from build123d import *

# Parameters (mm, degrees)
ESQUISSE1_W             = 90
ESQUISSE1_H             = 65
ESQUISSE1_R             = 7
ESQUISSE1_R_2           = 13
BOSS_EXTRU_1_DEPTH      = 8
ESQUISSE2_R             = 13
BOSS_EXTRU_2_DEPTH      = 3
ESQUISSE3_R             = 7
ESQUISSE3_R_2           = 1.5
ENL_V_MAT_EXTRU_1_DEPTH = 112.130553854
ESQUISSE4_R             = 8
ENL_V_MAT_EXTRU_2_DEPTH = 5.5
ESQUISSE5_W             = 45
ESQUISSE5_H             = 25
ENL_V_MAT_EXTRU_3_DEPTH = 112.30588484


with BuildPart() as part:
    # Esquisse1 → Boss.-Extru.1 (new body)
    with BuildSketch(Plane.XY):
        with Locations((45, 32.5)):
            Rectangle(ESQUISSE1_W, ESQUISSE1_H)
        with Locations((70, 20)):
            Circle(ESQUISSE1_R, mode=Mode.SUBTRACT)
        with Locations((17, 20)):
            Circle(ESQUISSE1_R_2, mode=Mode.SUBTRACT)
        with Locations((25, 48)):
            Circle(ESQUISSE1_R_2, mode=Mode.SUBTRACT)
    extrude(amount=BOSS_EXTRU_1_DEPTH)

    # Esquisse2 → Boss.-Extru.2 (add)
    with BuildSketch(Plane(origin=(0, 0, 0), x_dir=(-1, 0, 0), z_dir=(0, 0, -1))):
        with Locations((-17, 20)):
            Circle(ESQUISSE2_R)
    extrude(amount=-BOSS_EXTRU_2_DEPTH)

    # Esquisse3 → Enlèv. mat.-Extru.1 (cut, through all)
    with BuildSketch(Plane.XY.offset(3)):
        with Locations((17, 20)):
            Circle(ESQUISSE3_R)
        with Locations((27, 20)):
            Circle(ESQUISSE3_R_2)
        with Locations((17, 10)):
            Circle(ESQUISSE3_R_2)
        with Locations((7, 20)):
            Circle(ESQUISSE3_R_2)
        with Locations((17, 30)):
            Circle(ESQUISSE3_R_2)
    extrude(amount=-ENL_V_MAT_EXTRU_1_DEPTH, mode=Mode.SUBTRACT)

    # Esquisse4 → Enlèv. mat.-Extru.2 (cut)
    with BuildSketch(Plane.XY.offset(8)):
        with Locations((70, 20)):
            Circle(ESQUISSE4_R)
    extrude(amount=-ENL_V_MAT_EXTRU_2_DEPTH, mode=Mode.SUBTRACT)

    # Esquisse5 → Enlèv. mat.-Extru.3 (cut, through all)
    with BuildSketch(Plane.XY.offset(8)):
        with Locations((67.5, 52.5)):
            Rectangle(ESQUISSE5_W, ESQUISSE5_H)
    extrude(amount=-ENL_V_MAT_EXTRU_3_DEPTH, mode=Mode.SUBTRACT)


solid = part.part
Input: part model. Units: mm. Frame: model coordinates. A direction names the side the tool comes from. Give positions to 0.01 mm unless a question says otherwise; leave off trailing zeros. Write each loop counter-clockwise with the first axis right and the second up, starting at its lowest first coordinate (ties: lowest second). Pieces come first, ordered by that corner, then holes. Notation, with made-up numbers: M -2,72.5 L 18,72.5 A31 ccw 18,104.5 Z; hole C -34,35 d5. An arc over 180 degrees is marked long. Use one line per item in the form item = value.
1. Cut plane D-D on x = 27. Return loops of the section in (y, z).
Outcome:
outline = M 0,0 L 18.5,0 L 18.5,3 L 11.69,3 L 11.69,8 L 0,8 Z; M 21.5,0 L 35.15,0 L 35.15,8 L 28.31,8 L 28.31,3 L 21.5,3 Z; M 60.85,0 L 65,0 L 65,8 L 60.85,8 Z
2. Mould query, pull axis X, two halves, no side actions, for faces 4 (the face through (74, 14, 2.5)), 5 (the face through (22, 65, 4)), 6 (the face through (45, 52, 4)). Classes: released by +X, released by -X, zero draft, split by the parting line, or undercut.
Outcome:
face_4 = undercut
face_5 = zero draft
face_6 = released by +X
3. Ray query, L1, parallel to Y at x = 25, z = 2.5; L2, parallel to X at y = 48.5, z = 7.75; L3, parallel to Y at x = 27, z = 0.7. Return the intervals inside material, ascending.
Outcome:
L1 = 0 to 35, 61 to 65
L2 = 0 to 12.01, 37.99 to 45
L3 = 0 to 18.5, 21.5 to 35.15, 60.85 to 65
4. Reachability of faces 1 (the face through (44, 26, 8)), 2 (the face through (62, 20, 5)), 3 (the face through (67, 40, 4)) from +Z, -Z, +X, -X, +Y, -Y: full face, straight path, thin tool, end or side. Return the list, or none.
Outcome:
face_1 = +Z, +X, -X, +Y, -Y
face_2 = +Z
face_3 = +Z, -Z, +X, +Y
5. Cut plane C-C on y = 48. Return loops of the section in (x, z), and give its area (3 significant figures).
Outcome:
outline = M 0,0 L 12,0 L 12,8 L 0,8 Z; M 38,0 L 45,0 L 45,8 L 38,8 Z
area = 152 mm²
6. Cut plane A-A on z = 1. Return loops of the section in (x, y), and give its area (3 significant figures).
Outcome:
outline = M 0,0 L 90,0 L 90,40 L 45,40 L 45,65 L 0,65 Z; hole C 7,20 d3; hole C 17,20 d14; hole C 25,48 d26; hole C 17,10 d3; hole C 17,30 d3; hole C 27,20 d3; hole C 70,20 d14
area = 3,860 mm²
7. Cut plane B-B on x = 17. Return loops of the section in (y, z).
Outcome:
outline = M 0,0 L 8.5,0 L 8.5,3 L 7,3 L 7,8 L 0,8 Z; M 11.5,0 L 13,0 L 13,3 L 11.5,3 Z; M 27,0 L 28.5,0 L 28.5,3 L 27,3 Z; M 31.5,0 L 37.75,0 L 37.75,8 L 33,8 L 33,3 L 31.5,3 Z; M 58.25,0 L 65,0 L 65,8 L 58.25,8 Z
8. First-contact query: P1, Ø2.5, axis at y = 48.5, z = 2.5, coming from the +X side; P2, Ø13, axis at x = 69, y = 21.5, coming from the +Z side; P3, Ø1.8, axis at x = 27, y = 20, coming from the +Z side; P4, Ø4, axis at x = 17, y = 30, coming from the +Z side. Flat tips, straight axial feed; report the tip coordinate or a pass-through.
Outcome:
P1 = 45
P2 = 8
P3 = through
P4 = 3
